Geometry: final body of the model. Coordinates: model frame, mm. A direction names the side the tool comes from. Round coordinates to 2 decimals unless told otherwise and drop trailing zeros. Order: outer loops, then holes, each group sorted by start corner. A loop starts at its lowest first (then second) coordinate and runs counter-clockwise, first axis right, second up. Notation, with made-up numbers: (-21, 76.5) - (35, 76.5) arc R27 cw to (35, 103.5) - close; hole circle Ø3 at (-33.5, 86). An arc over 180 degrees is marked (long way). Put each result on its own line as item: value. Start each with the question number.
(1) Pin query (flat end, axial travel): P1, Ø13.5, axis at x = -70, y = 0, coming from the +Z side; P2, Ø4, axis at x = 2, z = 2, coming from the +Y side; P3, Ø2, axis at y = 21, z = 4, coming from the -X side; P4, Ø2, axis at y = 18, z = -1.5, coming from the +X side. Return the tip coordinate at first contact, or that it passes through.
(2) Section B-B (x = 14.5). Output: boundary loops of the cut face in (y, z).
(3) Material intervals for L1, parallel to Y at x = -70, z = 1; L2, parallel to Y at x = -53.5, z = -1.5; L3, parallel to Y at x = 11.5, z = 3.25, sorted ascending. Write a range as [from, to].
(4) Pull-direction query (X, two-part tool) for faces 4 (the face through (-77.493, 0.33, -0.07)), 5 (the face through (0.01, -0.82, 0.07)), 6 (the face through (-11, -3, -5)); classes: released by +X, released by -X, zero draft, split by the parting line, or undercut.
(5) Section A-A (y = 0). Output: boundary loops of the cut face in (x, z), and give its area (3 significant figures).
(6) Access query for faces 1 (the face through (-55, 10, 0)), 2 (the face through (38.761, -41.426, 0.07)), 3 (the face through (-55, -10, 0)). Directions: +Z, -Z, +X, -X, +Y, -Y. A direction counts if a zero-diameter tool reaches every point of the face in a straight line with its end or side. Return the directions, or none.
(7) Section D-D (x = -52). Output: boundary loops of the cut face in (y, z), and give its area (3 significant figures).
from build123d import *

# Parameters (mm, degrees)
SKETCH1_R           = 7.5
BOSS_EXTRUDE1_DEPTH = 5
FILLET2_R           = 5


with BuildPart() as part:
    # Sketch1 → Boss-Extrude1 (new, symmetric)
    with BuildSketch(Plane.XY):
        with BuildLine():
            Line((40, -50), (40, -40))
            ThreePointArc((40, -40), (0, 0), (40, 40))
            Line((40, 40), (40, 50))
            ThreePointArc((40, 50), (17.639320225, 44.72135955), (0, 30))
            ThreePointArc((0, 30), (-17.639320225, 15.27864045), (-40, 10))
            Line((-40, 10), (-70, 10))
            ThreePointArc((-70, 10), (-80, 0), (-70, -10))
            Line((-70, -10), (-40, -10))
            ThreePointArc((-40, -10), (-17.639320225, -15.27864045), (0, -30))
            ThreePointArc((0, -30), (17.639320225, -44.72135955), (40, -50))
        make_face()
        with Locations((-70, 0)):
            Circle(SKETCH1_R, mode=Mode.SUBTRACT)
    extrude(amount=BOSS_EXTRUDE1_DEPTH, both=True)

    # Fillet2
    fillet2_edges = [part.edges().sort_by_distance(p)[0] for p in [
        (40, -50, 0),
        (40, -40, 0),
        (40, 50, 0),
        (40, 40, 0),
    ]]
    fillet(fillet2_edges, radius=FILLET2_R - 0.0001)  # a hair under: the kernel refuses the full size


solid = part.part
Checks:
1. P1: passes through
1. P2: stops at y = 34.7
1. P3: stops at x = -10
1. P4: stops at x = 4.8
2. outline: (-43.01, -5) - (-30.82, -5) - (-30.82, 5) - (-43.01, 5) - close; (30.82, -5) - (43.01, -5) - (43.01, 5) - (30.82, 5) - close
3. L1: y = [-10, -7.5], [7.5, 10]
3. L2: y = [-10, 10]
3. L3: y = [-41.08, -28.07], [28.07, 41.08]
4. face 4: undercut
4. face 5: released by +X
4. face 6: zero draft
5. outline: (-80, -5) - (-77.5, -5) - (-77.5, 5) - (-80, 5) - close; (-62.5, -5) - (0, -5) - (0, 5) - (-62.5, 5) - close
5. area: 650 mm²
6. face 1: +Z, -Z, -X, +Y
6. face 2: +Z, -Z, +X
6. face 3: +Z, -Z, -X, -Y
7. outline: (-10, -5) - (10, -5) - (10, 5) - (-10, 5) - close
7. area: 200 mm²
